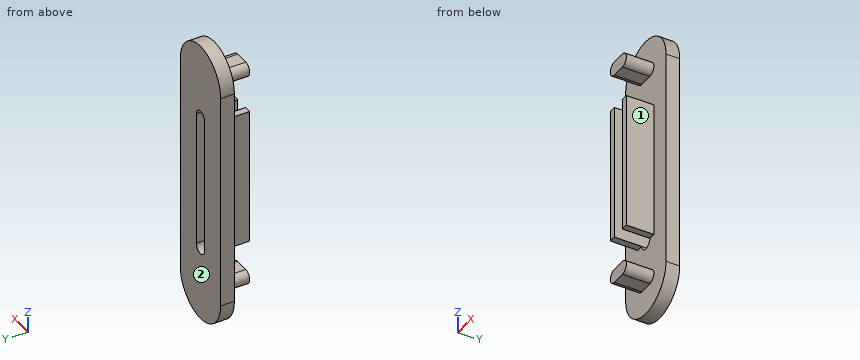
```python
from build123d import *

# Parameters (mm, degrees)
F1_DEPTH = 25.4
F3_DEPTH = 12.7
F4_W     = 6.35
F4_H     = 127
F5_DEPTH = 25.4


with BuildPart() as f1:
    # F0 (on Front) → F1 (new body)
    with BuildSketch(Plane.XZ):
        with BuildLine():
            Line((10.7133227866, 30.7250145495), (-1.9866772134, 30.7250145495))
            ThreePointArc((-1.9866772134, 30.7250145495), (-8.3366772134, 24.3750145495), (-1.9866772134, 18.0250145495))
            Line((-1.9866772134, 18.0250145495), (10.7133227866, 18.0250145495))
            ThreePointArc((10.7133227866, 18.0250145495), (17.0633227866, 24.3750145495), (10.7133227866, 30.7250145495))
        make_face()
    extrude(amount=F1_DEPTH)



with BuildPart() as f1b:
    # F0 (on Front) → F1, piece 2 (new body)
    with BuildSketch(Plane.XZ):
        with BuildLine():
            Line((10.7133227866, -172.4749854505), (-1.9866772134, -172.4749854505))
            ThreePointArc((-1.9866772134, -172.4749854505), (-8.3366772134, -178.8249854505), (-1.9866772134, -185.1749854505))
            Line((-1.9866772134, -185.1749854505), (10.7133227866, -185.1749854505))
            ThreePointArc((10.7133227866, -185.1749854505), (17.0633227866, -178.8249854505), (10.7133227866, -172.4749854505))
        make_face()
    extrude(amount=F1_DEPTH)


with BuildPart() as f1_1:
    add(f1.part)

    add(f1b.part)  # F3 merges F1b
    # F2 (on face) → F3 (join)
    with BuildSketch(Plane(origin=(0, 0, 0), x_dir=(-1, 0, 0), z_dir=(0, 1, 0))):
        with BuildLine():
            ThreePointArc((27.3866772134, 24.3750145495), (-4.3633227866, 56.1250145495), (-36.1133227866, 24.3750145495))
            Line((-36.1133227866, 24.3750145495), (-36.1133227866, -178.8249854505))
            ThreePointArc((-36.1133227866, -178.8249854505), (-4.3633227866, -210.5749854505), (27.3866772134, -178.8249854505))
            Line((27.3866772134, -178.8249854505), (27.3866772134, 24.3750145495))
        make_face()
        with BuildLine():
            Line((-10.7133227866, -140.7249854505), (-10.7133227866, -13.7249854505))
            ThreePointArc((-10.7133227866, -13.7249854505), (-4.3633227866, -7.3749854505), (1.9866772134, -13.7249854505))
            Line((1.9866772134, -13.7249854505), (1.9866772134, -140.7249854505))
            ThreePointArc((1.9866772134, -140.7249854505), (-4.3633227866, -147.0749854505), (-10.7133227866, -140.7249854505))
        make_face(mode=Mode.SUBTRACT)
    extrude(amount=F3_DEPTH)

    # F4 (on face) → F5 (join)
    with BuildSketch(Plane.XZ):
        with Locations((13.8883227866, -77.2249854505)):
            Rectangle(F4_W, F4_H)
        with Locations((-5.1616772134, -77.2249854505)):
            Rectangle(F4_W, F4_H)
    extrude(amount=F5_DEPTH)


solid = f1_1.part
```
Geometry check sheet. Reference: the model listing, model coordinates, mm. Face numbers are marked on the shaded views. A direction names the side the tool comes from. Give positions to 0.01 mm unless a question says otherwise; leave off trailing zeros. Loops run counter-clockwise (first coordinate to the right, second up) from the corner with the lowest first, then second, coordinate; pieces in that order, holes last. Notation, with made-up numbers: M 33,-1.5 L 89,-1.5 A21 ccw 89,16.5 Z; hole C 7.5,33.25 d11. An arc over 180 degrees is marked long. Answer as CSV lines item,"result".
Item 1: Cross-section at C-C on y = -21.5. Record the cut outline in (x, z).
Values:
outline,"M -8.34,-140.72 L -1.99,-140.72 L -1.99,-13.72 L -8.34,-13.72 Z; M -1.99,-185.17 L 10.71,-185.17 A6.35 ccw 10.71,-172.47 L -1.99,-172.47 A6.35 ccw Z; M -1.99,18.03 L 10.71,18.03 A6.35 ccw 10.71,30.73 L -1.99,30.73 A6.35 ccw Z; M 10.71,-140.72 L 17.06,-140.72 L 17.06,-13.72 L 10.71,-13.72 Z"
Item 2: Cross-section at A-A on z = -51.5. Record the cut outline in (x, y).
Values:
outline,"M -27.39,0 L -8.34,0 L -8.34,-25.4 L -1.99,-25.4 L -1.99,12.7 L -27.39,12.7 Z; M 10.71,-25.4 L 17.06,-25.4 L 17.06,0 L 36.11,0 L 36.11,12.7 L 10.71,12.7 Z"
Item 3: Access from +Z, -Z, +X, -X, +Y, -Y to the whole of each face (thin tool, end or side, straight path). Record for the marked faces 1 and 2.
Values:
face 1,"+Z, -Z, +X, -Y"
face 2,"+Z, -Z, +X, -X, +Y"
Item 4: Material ranges on line 1 (X direction, y = -0.5, z = -29.5); line 2 (X direction, y = 5.5, z = -114); line 3 (Z direction, x = -7.5, y = -15.5), recorded low to high.
Values:
line 1,"x = -8.34 to -1.99, 10.71 to 17.06"
line 2,"x = -27.39 to -1.99, 10.71 to 36.11"
line 3,"z = -181.98 to -175.67, -140.72 to -13.72, 21.22 to 27.53"
Item 5: Depth check by flat-ended pin: P1, Ø7, axis at x = -6, y = -18, coming from the +Z side; P2, Ø10, axis at x = 2.5, y = -13.5, coming from the -Z side (3 decimals); P3, Ø19, axis at x = 20, z = -11.5, coming from the -Y side; P4, Ø8, axis at x = 4, y = 8, coming from the -Z side (3 decimals). Enter the tip coordinate at first touch or a pass-through.
Values:
P1,"stops at z = 30.7"
P2,"stops at z = -185.175"
P3,"stops at y = -25.4"
P4,"stops at z = -210.575"
Item 6: Cross-section at B-B on y = 9. Record the cut outline in (x, z), and give its area (3 significant figures).
Values:
outline,"M -27.39,-178.82 A31.75 ccw 36.11,-178.82 L 36.11,24.38 A31.75 ccw -27.39,24.38 Z; hole M -1.99,-140.72 A6.35 ccw 10.71,-140.72 L 10.71,-13.72 A6.35 ccw -1.99,-13.72 Z"
area,"14,300 mm²"
Item 7: Cross-section at D-D on x = 13. Record the cut outline in (y, z).
Values:
outline,"M -25.4,-184.75 L 0,-184.75 L 0,-209.38 L 12.7,-209.38 L 12.7,54.93 L 0,54.93 L 0,30.3 L -25.4,30.3 L -25.4,18.45 L 0,18.45 L 0,-13.72 L -25.4,-13.72 L -25.4,-140.72 L 0,-140.72 L 0,-172.9 L -25.4,-172.9 Z"
